Autodesk Inventor part; units mm, degrees
ref_plane "YZ Plane" through (0, 0, 0) normal (1, 0, 0) x (0, 1, 0)
ref_plane "XZ Plane" through (0, 0, 0) normal (0, 1, 0) x (-1, 0, 0)
ref_plane "XY Plane" through (0, 0, 0) normal (0, 0, 1) x (1, 0, 0)
sketch "Skizze1" plane through (0, 0, 0) normal (0, 1, 0) x (-1, 0, 0)
  arc A0 (-116, -64) -> (-114, -66) centre (-114, -64) ccw
  arc A1 (-114, -62) -> (-112, -64) centre (-112, -62) ccw
  line L0 (-114, -62) -> (-114, 62)
  line L1 (-116, 64) -> (-116, -64)
  line L2 (-120, -65) -> (-120, 65)
  line L3 (112, -64) -> (-112, -64)
  line L4 (-114, -66) -> (114, -66)
  line L5 (115, -70) -> (-115, -70)
  line L6 (-112, 64) -> (112, 64)
  line L7 (114, 64) -> (-114, -64) construction
  line L8 (114, 66) -> (-114, 66)
  line L9 (-116, 66) -> (116, -66) construction
  line L10 (-116, -66) -> (116, 66) construction
  line L11 (-115, 70) -> (115, 70)
  line L12 (120, 70) -> (-120, -70) construction
  line L13 (120, -70) -> (-120, 70) construction
  line L14 (114, -64) -> (-114, 64) construction
  line L15 (120, 65) -> (120, -65)
  arc A2 (-120, -65) -> (-115, -70) centre (-115, -65) ccw
  arc A3 (-112, 64) -> (-114, 62) centre (-112, 62) ccw
  arc A4 (-115, 70) -> (-120, 65) centre (-115, 65) ccw
  arc A5 (-114, 66) -> (-116, 64) centre (-114, 64) ccw
  arc A6 (120, 65) -> (115, 70) centre (115, 65) ccw
  arc A7 (115, -70) -> (120, -65) centre (115, -65) ccw
  line L16 (116, -64) -> (116, 64)
  arc A8 (114, -66) -> (116, -64) centre (114, -64) ccw
  arc A9 (112, -64) -> (114, -62) centre (112, -62) ccw
  line L17 (114, 62) -> (114, -62)
  arc A10 (114, 62) -> (112, 64) centre (112, 62) ccw
  arc A11 (116, 64) -> (114, 66) centre (114, 64) ccw
  line L18 (-160, -110) -> (160, -110)
  line L19 (160, -110) -> (160, 110)
  line L20 (160, 110) -> (-160, 110)
  line L21 (-160, 110) -> (-160, -110)
  line L22 (-160, -110) -> (160, 110) construction
  line L23 (160, -110) -> (-160, 110) construction
  circle A12 centre (-140, -90) radius 2.75
  line L24 (140, 90) -> (-140, 90)
  line L25 (-140, 90) -> (-140, -90)
  line L26 (-140, -90) -> (140, -90)
  line L27 (140, -90) -> (140, 90)
  line L28 (140, 90) -> (-140, -90) construction
  line L29 (-140, 90) -> (140, -90) construction
  circle A13 centre (140, -90) radius 2.75
  circle A14 centre (140, 90) radius 2.75
  circle A15 centre (-140, 90) radius 2.75
  point P0 (0, 0)
  point P1 (0, 0)
  point P2 (0, 0)
  point P3 (0, 0)
  point P4 (0, 0)
  point P5 (0, 0)
  point P6 (0, 0)
  dimension "d0" = 140
  dimension "d1" = 240
  dimension "d2" = 5
  dimension "d3" = 232
  dimension "d4" = 132
  dimension "d5" = 2
  dimension "d6" = 128
  dimension "d7" = 228
  dimension "d8" = 2
  dimension "d19" = 40
  dimension "d20" = 40
  dimension "d21" = 5.5
  dimension "d23" = 20
  dimension "d24" = 20
extrude "Extrusion1" add sketch "Skizze1" along normal blind 6 contours L21 L20 L19 L18 | L26 L25 A12 | A12 L25 L26 | A12 L25 A15 L24 A14 L27 A13 L26 | A13 L27 L26 | L26 L27 A13 | A15 L24 L25 | L25 L24 A15 | A14 L24 L27 | L27 L24 A14
extrude "Extrusion2" add sketch "Skizze1" against normal blind 6 contours L2 A4 L11 A6 L15 A7 L5 A2 | L21 L20 L19 L18 | L26 L25 A12 | A12 L25 L26 | A12 L25 A15 L24 A14 L27 A13 L26 | A13 L27 L26 | L26 L27 A13 | A15 L24 L25 | L25 L24 A15 | A14 L24 L27 | L27 L24 A14
extrude "Extrusion3" cut sketch "Skizze1" along normal through all both and the other way through all contours L26 L25 A12 | A12 L25 L26 | A13 L27 L26 | L26 L27 A13 | A15 L24 L25 | L25 L24 A15 | A14 L24 L27 | L27 L24 A14
equation "\"d14\" = mdf_thickness"
equation "\"d16\" = mdf_thickness"
equation "\"d10\" = 6"
equation "\"kg_thickness\" = 4.9"
equation "\"ht_thickness\" = 1.9"
equation "\"case_thickness\" = 18"
equation "\"inner_thickness\" = 15"
equation "\"gap_fit\" = 0.1"
equation "\"gap_slide\" = 0.2"
equation "\"gap_air\" = 1"
equation "\"bore_diameter\" = 73"
equation "\"mdf_thickness\" = 6"
equation "\"tape_width\" = 15"
equation "\"tape_thickness\" = 3"
equation "\"inner_depth\" = 255"
properties part number "Flachfilter_Rahmen"
Model file for the job. Use its own axes, mm. A direction names the side the tool comes from. Give positions to 0.01 mm unless a question says otherwise; leave off trailing zeros. Write each loop counter-clockwise with the first axis right and the second up, starting at its lowest first coordinate (ties: lowest second). Pieces come first, ordered by that corner, then holes. Notation, with made-up numbers: M -14.5,5.5 L -3.5,5.5 A18 cw -3.5,18.5 Z; hole C -17,47 d11. An arc over 180 degrees is marked long. Use a Markdown table: item, result.
1) Drill centre lines: line 1 (Z direction, x = 140, y = 1); line 2 (X direction, y = -2.5, z = -12.5); line 3 (Z direction, x = -103, y = 3.75). Where is each one in solid material? Low to high. Write a range as from..to.
Responses:
| item | result |
|---|---|
| line 1 | z = -110..-92.75, -87.25..87.25, 92.75..110 |
| line 2 | x = -160..-116, 116..160 |
| line 3 | z = -110..-70, 70..110 |
2) Pin check, flat tip, straight feed: pin 1 (6.5 mm diameter, centred on x = -140, z = -90, fed in from -Y). Stop position of the tip, or through.
Responses:
| item | result |
|---|---|
| pin 1 | stops at y = -6 |
3) Cut at B-B (x = -4). List the corners of the cut face in (y, z), and give its area (3 significant figures).
Responses:
| item | result |
|---|---|
| outline | M -6,-110 L 6,-110 L 6,-70 L 0,-70 L 0,-66 L -6,-66 Z; M -6,66 L 0,66 L 0,70 L 6,70 L 6,110 L -6,110 Z |
| area | 1,010 mm2 |
4) Cut at C-C (y = 3). List the corners of the cut face in (x, z), and give its area (3 significant figures).
Responses:
| item | result |
|---|---|
| outline | M -160,-110 L 160,-110 L 160,110 L -160,110 Z; hole C -140,-90 d5.5; hole C -140,90 d5.5; hole M -120,-65 A5 ccw -115,-70 L 115,-70 A5 ccw 120,-65 L 120,65 A5 ccw 115,70 L -115,70 A5 ccw -120,65 Z; hole C 140,-90 d5.5; hole C 140,90 d5.5 |
| area | 36,700 mm2 |
5) Tool access for faces 1 (the flat face through (120, 3, -1)), 2 (the flat face through (2, -6, 75)), 3 (the flat face through (2, -3, -66)): list every direction of +Z, -Z, +X, -X, +Y, -Y with a clear straight run to the whole face (end or side of a thin tool).
Responses:
| item | result |
|---|---|
| face 1 | +Y |
| face 2 | +Z, -Z, +X, -X, -Y |
| face 3 | +Y, -Y |
6) Pull direction Z, two halves, no side cores. Call faces 4 (the flat face through (2, 6, 75)), 5 (the flat face through (2, 0, -110)), 6 (the flat face through (36, 0, -67)): +Z half, -Z half, draft (parallel to the pull), parting line (faces both ways), or undercut.
Responses:
| item | result |
|---|---|
| face 4 | draft |
| face 5 | -Z half |
| face 6 | undercut |
7) Cut at A-A (z = 32). List the corners of the cut face in (x, y).
Responses:
| item | result |
|---|---|
| outline | M -160,-6 L -116,-6 L -116,0 L -120,0 L -120,6 L -160,6 Z; M 116,-6 L 160,-6 L 160,6 L 120,6 L 120,0 L 116,0 Z |
